from build123d import *

# Parameters (mm, degrees)
SKETCH1_R           = 1.5
BOSS_EXTRUDE2_DEPTH = 2
SKETCH3_R           = 12
BOSS_EXTRUDE3_DEPTH = 2
SKETCH4_R           = 0.5
SKETCH5_R           = 2
BOSS_EXTRUDE4_DEPTH = 4.040735944
FILLET1_R           = 1
SKETCH7_R           = 12
CUT_EXTRUDE3_DEPTH  = 0.6


with BuildPart() as part:
    # Sketch1 → Boss-Extrude2 (new body)
    with BuildSketch(Plane(origin=(0, 0, 0), x_dir=(1, 0, 0), z_dir=(0, 1, 0))):
        with BuildLine():
            Line((-15.5, 15), (15.5, 15))
            ThreePointArc((15.5, 15), (16.914213562, 14.414213562), (17.5, 13))
            Line((17.5, 13), (17.5, -13))
            ThreePointArc((17.5, -13), (16.914213562, -14.414213562), (15.5, -15))
            Line((15.5, -15), (-15.5, -15))
            ThreePointArc((-15.5, -15), (-16.914213562, -14.414213562), (-17.5, -13))
            Line((-17.5, -13), (-17.5, 13))
            ThreePointArc((-17.5, 13), (-16.914213562, 14.414213562), (-15.5, 15))
        make_face()
        with Locations(Location((-14.79625841, 12.682507209, 0), (0, 0, 270))):
            Circle(SKETCH1_R, mode=Mode.SUBTRACT)
        with Locations(Location((-14.79625841, -12.682507209, 0), (0, 0, 270))):
            Circle(SKETCH1_R, mode=Mode.SUBTRACT)
        with Locations(Location((14.79625841, 12.682507209, 0), (0, 0, 270))):
            Circle(SKETCH1_R, mode=Mode.SUBTRACT)
        with Locations(Location((14.79625841, -12.682507209, 0), (0, 0, 270))):
            Circle(SKETCH1_R, mode=Mode.SUBTRACT)
    extrude(amount=BOSS_EXTRUDE2_DEPTH)

    # Sketch3 → Boss-Extrude3 (add)
    with BuildSketch(Plane.XZ):
        with Locations(Location((0, 0, 0), (0, 0, 90))):
            Circle(SKETCH3_R)
    extrude(amount=BOSS_EXTRUDE3_DEPTH)

    # Sketch4 → Revolve1 (revolve)
    with BuildSketch(Plane(origin=(0, 0, 0), x_dir=(0, 0, -1), z_dir=(1, 0, 0))):
        with Locations((-12, -1.5)):
            Circle(SKETCH4_R)
    revolve(axis=Axis((0, 0, 0), (0, -1, 0)))

    # Sketch5 → Boss-Extrude4 (add)
    with BuildSketch(Plane.XZ.offset(2)):
        with Locations(Location((0, 0, 0), (0, 0, 270))):
            Circle(SKETCH5_R)
    extrude(amount=BOSS_EXTRUDE4_DEPTH)

    # Fillet1
    fillet1_edges = [part.edges().sort_by_distance(p)[0] for p in [
        (0, -6.040735944, 2),
    ]]
    fillet(fillet1_edges, radius=FILLET1_R)

    # Sketch7 → Cut-Extrude3 (cut)
    with BuildSketch(Plane(origin=(0, 2, 0), x_dir=(1, 0, 0), z_dir=(0, 1, 0))):
        with Locations(Location((0, 0, 0), (0, 0, 270))):
            Circle(SKETCH7_R)
    extrude(amount=-CUT_EXTRUDE3_DEPTH, mode=Mode.SUBTRACT)


solid = part.part
Input: part model. Units: mm. Frame: model coordinates. A direction names the side the tool comes from. Give positions to 0.01 mm unless a question says otherwise; leave off trailing zeros. Loops run counter-clockwise (first coordinate to the right, second up) from the corner with the lowest first, then second, coordinate; pieces in that order, holes last. Notation, with made-up numbers: (-16.75, 76.25) -> (1.25, 76.25) arc R22 ccw to (1.25, 94.25) -> close; hole circle Ø4 at (41, 44.5). An arc over 180 degrees is marked (long way). Answer as a JSON object with one key per item and string values. Group by question number.
Item 1: Cut plane A-A, the plane y = 0.5. Return the cut outline in (x, z).
Item 2: Pull-direction query (X, two-part tool) for faces 1 (the cylindrical face through (-16.9, 0.99, 14.43)), 2 (the cylindrical face through (-16.127, 0.986, -11.99)), 3 (the cylindrical face through (15.247, 0.986, -11.252)), 4 (the cylindrical face through (-3.604, -0.493, 11.446)); classes: released by +X, released by -X, zero draft, split by the parting line, or undercut.
Item 3: Cut plane B-B, the plane y = -4.5. Return the cut outline in (x, z), and give its area (3 significant figures).
Item 4: Pin query (flat end, axial travel): P1, Ø2, axis at x = -9, z = 5, coming from the -Y side; P2, Ø1.5, axis at x = 0, y = -3.5, coming from the +Z side; P3, Ø7, axis at x = -2, z = -2.5, coming from the +Y side. Return the tip coordinate at first contact, or that it passes through.
Item 5: Reachability of faces 5 (the cylindrical face through (-2, -3, 0)), 6 (the cylindrical face through (3.604, 1.704, 11.446)), 7 (the flat face through (12, 2, 3)) from +Z, -Z, +X, -X, +Y, -Y: full face, straight path, thin tool, end or side. Return the list, or none.
Item 6: Line query: probe 1 along Y at (x, z) = (-3.5, 13.25); probe 2 along X at (y, z) = (1.75, -5.5); probe 3 along Y at (x, z) = (7.5, -9.75). Output: solid intervals per line, ascending.
Checks:
{
 "1": {"outline": "(-17.5, -13) arc R2 ccw to (-15.5, -15) -> (15.5, -15) arc R2 ccw to (17.5, -13) -> (17.5, 13) arc R2 ccw to (15.5, 15) -> (-15.5, 15) arc R2 ccw to (-17.5, 13) -> close; hole circle Ø3 at (-14.8, -12.68); hole circle Ø3 at (-14.8, 12.68); hole circle Ø3 at (14.8, -12.68); hole circle Ø3 at (14.8, 12.68)"},
 "2": {"face 1": "released by -X", "face 2": "undercut", "face 3": "undercut", "face 4": "split by the parting line"},
 "3": {"outline": "circle Ø4 at (0, 0)", "area": "12.6 mm²"},
 "4": {"P1": "stops at y = -2", "P2": "stops at z = 2", "P3": "stops at y = 1.4"},
 "5": {"face 5": "-Y", "face 6": "+Y", "face 7": "+Z, -Z, +X, -X, +Y"},
 "6": {"probe 1": "y = 0 to 2", "probe 2": "x = -17.5 to -10.67, 10.67 to 17.5", "probe 3": "y = -1.9 to -1.1, 0 to 2"}
}
